from build123d import *

# Parameters (mm, degrees)
F1_DEPTH = 5
F2_R     = 5
F3_R     = 5


with BuildPart() as f1:
    # F0 (on Top) → F1 (new body)
    with BuildSketch(Plane.XY):
        Polygon((-55, -30), (-55, -50), (55, -50), (55, -30), (50, -30), (50, -15), (55, -15), (55, 15), (50, 15), (50, 30), (55, 30), (55, 50), (30, 50), (30, 45), (15, 45), (15, 50), (-15, 50), (-15, 45), (-30, 45), (-30, 50), (-55, 50), (-55, 30), (-50, 30), (-50, 15), (-55, 15), (-55, -15), (-50, -15), (-50, -30), align=None)
        Polygon((-40.201199, -29.78924), (-40.201199, 29.78924), (-7.433034, 0), align=None, mode=Mode.SUBTRACT)
        Polygon((0, -6.757304), (32.768164, -36.546544), (-32.768164, -36.546544), align=None, mode=Mode.SUBTRACT)
        Polygon((-32.768164, 36.546544), (32.768164, 36.546544), (0, 6.757304), align=None, mode=Mode.SUBTRACT)
        Polygon((7.433034, 0), (40.201199, 29.78924), (40.201199, -29.78924), align=None, mode=Mode.SUBTRACT)
    extrude(amount=F1_DEPTH)

    # F2
    f2_edges = [f1.edges().sort_by_distance(p)[0] for p in [
        (55, 50, 2.5),
        (-55, 50, 2.5),
    ]]
    fillet(f2_edges, radius=F2_R)

    # F3
    f3_edges = [f1.edges().sort_by_distance(p)[0] for p in [
        (55, -50, 2.5),
        (-55, -50, 2.5),
    ]]
    fillet(f3_edges, radius=F3_R)


solid = f1.part
The listing builds one solid part. Answer for the finished solid, in the listing's coordinates (mm). A direction names the side the tool comes from. Give positions to 0.01 mm unless a question says otherwise; leave off trailing zeros. Write each loop counter-clockwise with the first axis right and the second up, starting at its lowest first coordinate (ties: lowest second). Pieces come first, ordered by that corner, then holes.
1) Given P1, Ø2.5, axis at y = 23, z = 3.5, coming from the +X side; P2, Ø1.5, axis at x = 52.5, z = 2.5, coming from the -Y side; P3, Ø8, axis at x = 35, y = -11.5, coming from the +Z side; P4, Ø1.5, axis at x = 53, z = 3.5, coming from the +Y side, each flat-ended and moving along its own axis, determine where each tip first touches the part or whether it passes through.
2) A tool of negligible diameter and unlimited length cuts with its end or side. For faces 4 (the face through (-50, -22, 2)), 5 (the face through (50, -23, 2)), 6 (the face through (-16.15, 21.44, 2.46)), 7 (the face through (-1, -50, 2)), 8 (the face through (30, 48, 2)), from which of +Z, -Z, +X, -X, +Y, -Y can it reach the whole face along a straight path? Write none if from no direction.
3) Find the intervals of material crossed by L1, parallel to X at y = -2, z = 0.35; L2, parallel to X at y = -17, z = 4.15; L3, parallel to X at y = 46.5, z = 2.65, in increasing order.
4) Section C-C (y = 22) is taken. Write down the section's boundary in (x, z).
5) Section A-A (x = 20) is taken. Write down the section's boundary in (y, z).
6) Section D-D (x = 2) is taken. Write down the section's boundary in (y, z), and give its area (3 significant figures).
7) Section B-B (x = 36.5) is taken. Write down the section's boundary in (y, z).
8) For a pull along X with two mould halves and no side action, classify faces 1 (the face through (0, 36.547, 2)), 2 (the face through (-54, 48, 3)), 3 (the face through (53, -49, 3)) as pulls with the +X half, pulls with the -X half, needs draft (parallel to the pull), parting line crosses it, or undercut.
Response:
1. P1: stops at x = 50
1. P2: stops at y = -49.68
1. P3: passes through
1. P4: stops at y = 49.47
2. face 4: +Z, -Z, -X
2. face 5: +Z, -Z, +X
2. face 6: +Z, -Z
2. face 7: +Z, -Z, +X, -X, -Y
2. face 8: +Z, -Z, +Y
3. L1: x = -55 to -40.2, -9.63 to 9.63, 40.2 to 55
3. L2: x = -50 to -40.2, -26.13 to -11.27, 11.27 to 26.13, 40.2 to 50
3. L3: x = -54.77 to -30, -15 to 15, 30 to 54.77
4. outline: (-50, 0) - (-40.2, 0) - (-40.2, 5) - (-50, 5) - close; (-31.63, 0) - (-16.77, 0) - (-16.77, 5) - (-31.63, 5) - close; (16.77, 0) - (31.63, 0) - (31.63, 5) - (16.77, 5) - close; (40.2, 0) - (50, 0) - (50, 5) - (40.2, 5) - close
5. outline: (-50, 0) - (-36.55, 0) - (-36.55, 5) - (-50, 5) - close; (-24.94, 0) - (-11.42, 0) - (-11.42, 5) - (-24.94, 5) - close; (11.42, 0) - (24.94, 0) - (24.94, 5) - (11.42, 5) - close; (36.55, 0) - (45, 0) - (45, 5) - (36.55, 5) - close
6. outline: (-50, 0) - (-36.55, 0) - (-36.55, 5) - (-50, 5) - close; (-8.58, 0) - (8.58, 0) - (8.58, 5) - (-8.58, 5) - close; (36.55, 0) - (50, 0) - (50, 5) - (36.55, 5) - close
6. area: 220 mm2
7. outline: (-50, 0) - (-26.42, 0) - (-26.42, 5) - (-50, 5) - close; (26.42, 0) - (50, 0) - (50, 5) - (26.42, 5) - close
8. face 1: undercut
8. face 2: pulls with the -X half
8. face 3: pulls with the +X half
